Drawing for the job (mm, zero at the part's lowest x, y, z). A direction names the side the tool comes from. Coordinates: 2 decimals unless noted, no trailing zeros. Loops run counter-clockwise (first coordinate to the right, second up) from the corner with the lowest first, then second, coordinate; pieces in that order, holes last. Notation, with made-up numbers: (77, 8.25) - (133, 8.25) arc R14 cw to (133, 20.25) - close; hole circle Ø2 at (19, 77.25). An arc over 180 degrees is marked (long way). Put each result on its own line as item: value.
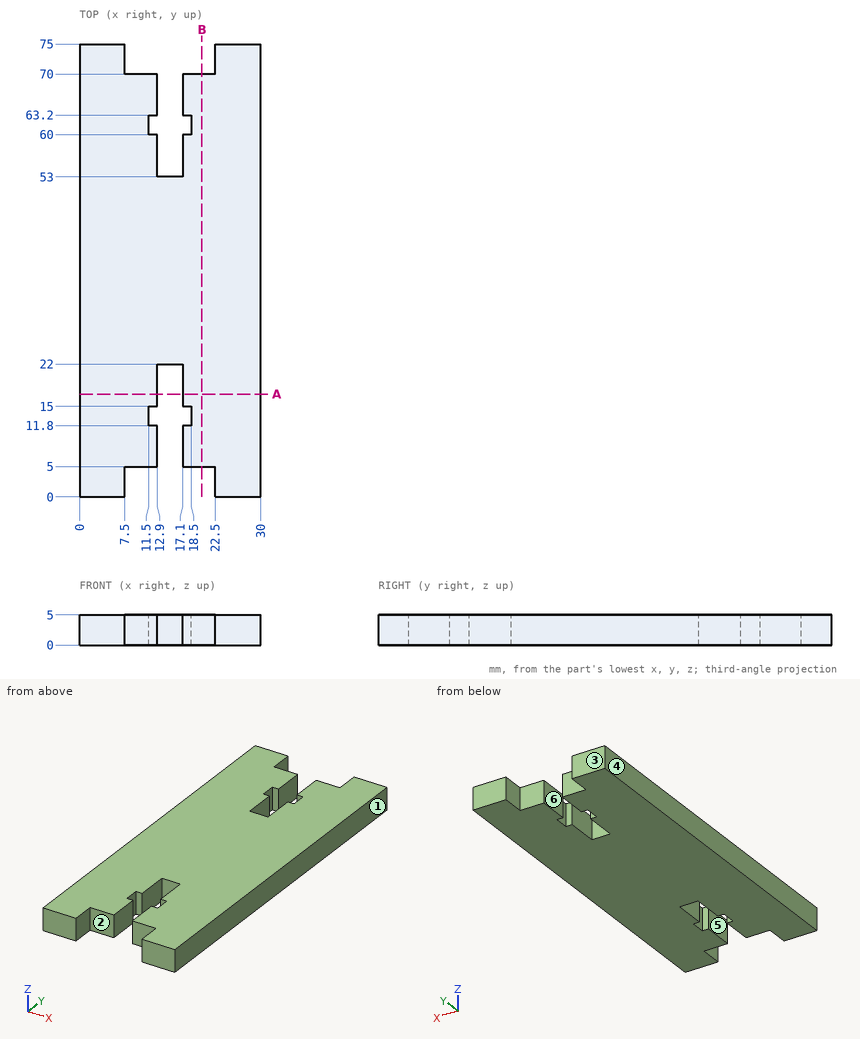
Q1. Pin check, flat tips, straight feed: pin 1 Ø1.3 at (x, z) = (14, 3) entering from +Y; pin 2 Ø1.1 at (x, z) = (17.5, 2) entering from +Y; pin 3 Ø1.1 at (x, z) = (17.5, 1.5) entering from -Y. Stop position of each tip, or through.
Determined:
pin 1: y = 53
pin 2: y = 70
pin 3: y = 5
Q2. Mould opens along X. For the marked faces 1, 2 and 3 say: +X half, -X half, draft (parallel to the pull), parting line (faces both ways), or undercut.
Determined:
face 1: +X half
face 2: undercut
face 3: draft
Q3. Slice it at A-A, the plane y = 17. Give the cut face in (x, z), then the cut area to 3 significant figures.
Determined:
outline: (0, 0) - (12.9, 0) - (12.9, 5) - (0, 5) - close; (17.1, 0) - (30, 0) - (30, 5) - (17.1, 5) - close
area: 129 mm2
Q4. Slice it at B-B, the plane x = 20.25. Give the cut face in (y, z), then the cut area to 3 significant figures.
Determined:
outline: (5, 0) - (70, 0) - (70, 5) - (5, 5) - close
area: 325 mm2
Q5. Tool access for the marked faces 4, 5 and 6: list every direction of +Z, -Z, +X, -X, +Y, -Y with a clear straight run to the whole face (end or side of a thin tool).
Determined:
face 4: +Z, -Z, -X, +Y, -Y
face 5: +Z, -Z, -Y
face 6: +Z, -Z, +Y
Q6. Wall check: L1, parallel to Y at x = 12, z = 4.05; L2, parallel to X at y = 8, z = 2.5; L3, parallel to X at y = 12.5, z = 4.4. Give the ranges that are in metal, low to high. Write a range as from..to.
Determined:
L1: 5..11.8, 15..60, 63.2..70
L2: 0..12.9, 17.1..30
L3: 0..11.5, 18.5..30
